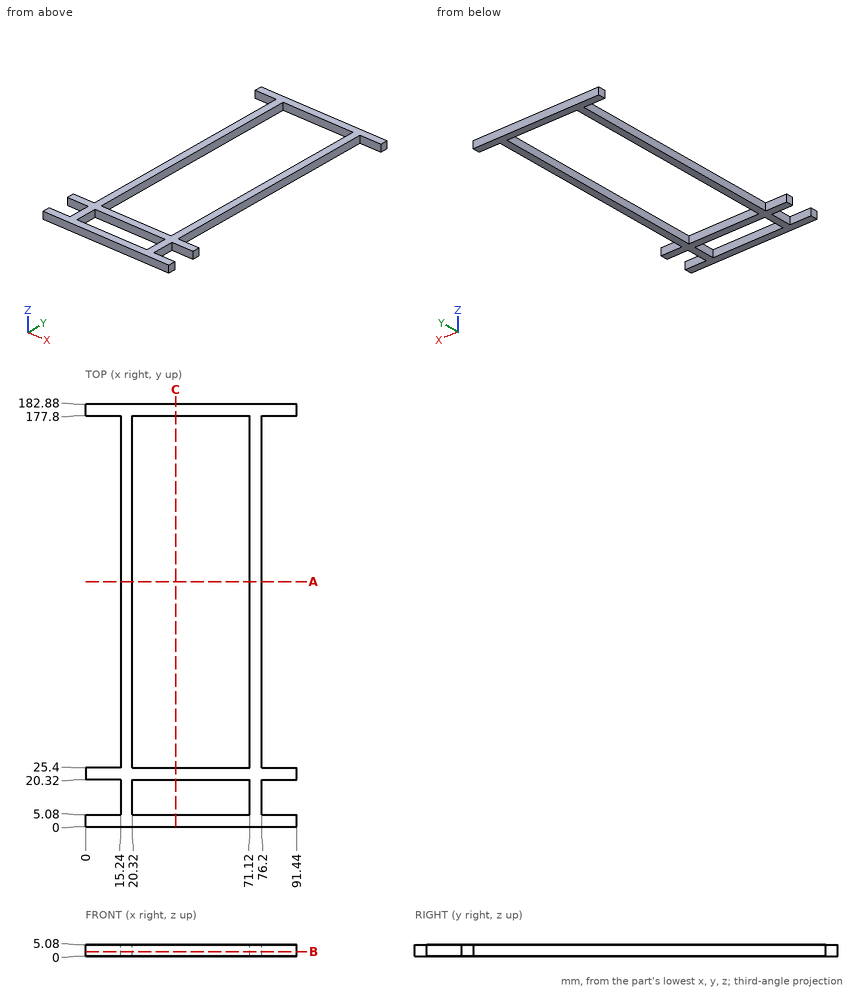
Print and shaded views of the part. All mm, measured from the part's lowest x, y and z. Coordinates: 2 decimals unless noted, no trailing zeros. Loops run counter-clockwise (first coordinate to the right, second up) from the corner with the lowest first, then second, coordinate; pieces in that order, holes last. Notation, with made-up numbers: (86, -34.75) - (91, -34.75) arc R34 cw to (91, -2.75) - close; hole circle Ø8 at (51, 13.25). An arc over 180 degrees is marked (long way). Write item = value, one per line. Start each with the question number.
Item 1: Wall check: L1, parallel to Y at x = 22.5, z = 3.8; L2, parallel to X at y = 69.5, z = 1.1. Give the ranges that are in metal, low to high. Write a range as from..to.
Item 2: Flat gauge pin, fed straight in: pin 1 Ø2.5 at (y, z) = (10, 2.5) entering from +X. Where does the tip first touch, or does it go through?
Item 3: Cut at B-B, the plane z = 2.1. Give the cut face in (x, y).
Item 4: Cut at C-C, the plane x = 39. Give the cut face in (y, z).
Item 5: Cut at A-A, the plane y = 106. Give the cut face in (x, z).
The answers:
q1.L1 = 0..5.08, 20.32..25.4, 177.8..182.88
q1.L2 = 15.24..20.32, 71.12..76.2
q2.pin_1 = 76.2
q3.outline = (0, 0) - (91.44, 0) - (91.44, 5.08) - (76.2, 5.08) - (76.2, 20.32) - (91.44, 20.32) - (91.44, 25.4) - (76.2, 25.4) - (76.2, 177.8) - (91.44, 177.8) - (91.44, 182.88) - (0, 182.88) - (0, 177.8) - (15.24, 177.8) - (15.24, 25.4) - (0, 25.4) - (0, 20.32) - (15.24, 20.32) - (15.24, 5.08) - (0, 5.08) - close; hole (20.32, 5.08) - (71.12, 5.08) - (71.12, 20.32) - (20.32, 20.32) - close; hole (20.32, 25.4) - (71.12, 25.4) - (71.12, 177.8) - (20.32, 177.8) - close
q4.outline = (0, 0) - (5.08, 0) - (5.08, 5.08) - (0, 5.08) - close; (20.32, 0) - (25.4, 0) - (25.4, 5.08) - (20.32, 5.08) - close; (177.8, 0) - (182.88, 0) - (182.88, 5.08) - (177.8, 5.08) - close
q5.outline = (15.24, 0) - (20.32, 0) - (20.32, 5.08) - (15.24, 5.08) - close; (71.12, 0) - (76.2, 0) - (76.2, 5.08) - (71.12, 5.08) - close
